Verification items for the finished model (mm, model axes). A direction names the side the tool comes from. Coordinates: 2 decimals unless noted, no trailing zeros. Order: outer loops, then holes, each group sorted by start corner. A loop starts at its lowest first (then second) coordinate and runs counter-clockwise, first axis right, second up. Notation, with made-up numbers: M 48,83 L 105,83 A11 ccw 105,90 Z; hole C 88,70 d4. An arc over 180 degrees is marked long. Return JSON: item names as keys, results as strings.
```python
from build123d import *

# Parameters (mm, degrees)
F1_DEPTH = 30
F2_R     = 2.25
F3_DEPTH = 25
F5_DEPTH = 4
F6_SIZE  = 5


with BuildPart() as f1:
    # F0 (on Top) → F1 (new body)
    with BuildSketch(Plane.XY):
        with BuildLine():
            ThreePointArc((6.4, 16.018817), (0, -17.25), (-6.4, 16.018817))
            Line((-6.4, 16.018817), (-6.4, 22.25))
            Line((-6.4, 22.25), (-44.75, 22.25))
            Line((-44.75, 22.25), (-44.75, 14.25))
            Line((-44.75, 14.25), (-22.25, 14.25))
            Line((-22.25, 14.25), (-22.25, 0))
            ThreePointArc((-22.25, 0), (0, -22.25), (22.25, 0))
            Line((22.25, 0), (22.25, 14.25))
            Line((22.25, 14.25), (44.75, 14.25))
            Line((44.75, 14.25), (44.75, 22.25))
            Line((44.75, 22.25), (6.4, 22.25))
            Line((6.4, 22.25), (6.4, 16.018817))
        make_face()
    extrude(amount=F1_DEPTH)

    # F2 (on face) → F3 (cut)
    with BuildSketch(Plane.XZ.offset(-14.25)):
        with Locations((-34.75, 22.5)):
            Circle(F2_R)
        with Locations((-34.75, 7.5)):
            Circle(F2_R)
        with Locations((34.75, 22.5)):
            Circle(F2_R)
        with Locations((34.75, 7.5)):
            Circle(F2_R)
    extrude(amount=-F3_DEPTH, mode=Mode.SUBTRACT)

    # F4 (on face) → F5 (cut)
    with BuildSketch(Plane.XZ.offset(-14.25)):
        Polygon((-30.525, 20.060695), (-30.525, 24.939305), (-34.75, 27.37861), (-38.975, 24.939305), (-38.975, 20.060695), (-34.75, 17.62139), align=None)
        Polygon((-30.525, 5.060695), (-30.525, 9.939305), (-34.75, 12.37861), (-38.975, 9.939305), (-38.975, 5.060695), (-34.75, 2.62139), align=None)
        Polygon((38.975, 5.060695), (38.975, 9.939305), (34.75, 12.37861), (30.525, 9.939305), (30.525, 5.060695), (34.75, 2.62139), align=None)
        Polygon((34.75, 27.37861), (30.525, 24.939305), (30.525, 20.060695), (34.75, 17.62139), (38.975, 20.060695), (38.975, 24.939305), align=None)
    extrude(amount=-F5_DEPTH, mode=Mode.SUBTRACT)

    # F6
    f6_edges = [f1.edges().sort_by_distance(p)[0] for p in [
        (-22.25, 14.25, 15),
        (22.25, 14.25, 15),
    ]]
    chamfer(f6_edges, length=F6_SIZE)


solid = f1.part
```
Q1. Go/stop test with flat-tipped pins: pin 1 (1.5 mm diameter, centred on y = 13, z = 16.5, fed in from -X); pin 2 (5 mm diameter, centred on y = 8.5, z = 10, fed in from +X); pin 3 (1 mm diameter, centred on x = -26.5, z = 11, fed in from -Y). Record where each tip stops, or that it passes through.
Values:
{"pin 1": "x = -26.75", "pin 2": "x = 24", "pin 3": "y = 13"}
Q2. Cross-section at D-D, the plane z = 14.75. Record the boundary of the cut face in (x, y), and give its area (3 significant figures).
Values:
{"outline": "M -44.75,14.25 L -27.25,14.25 L -22.25,9.25 L -22.25,0 A22.25 ccw 22.25,0 L 22.25,9.25 L 27.25,14.25 L 44.75,14.25 L 44.75,22.25 L 6.4,22.25 L 6.4,16.02 A17.25 cw long -6.4,16.02 L -6.4,22.25 L -44.75,22.25 Z", "area": "1,150 mm^2"}
Q3. Draft check along X on faces 1 (the face through (-33.712, 20.222, 20.504)), 2 (the face through (44.75, 18, 15)), 3 (the face through (9, 15, 0)). Enter one of: pulls with the +X half, pulls with the -X half, needs draft (parallel to the pull), parting line crosses it, or undercut.
Values:
{"face 1": "undercut", "face 2": "pulls with the +X half", "face 3": "needs draft"}
Q4. Cross-section at A-A, the plane z = 7.5. State how many separate pieces and enclosed holes the cut face has, and give its area (3 significant figures).
Values:
{"separate pieces": "3", "enclosed holes": "0", "area": "1,050 mm^2"}
Q5. Cross-section at C-C, the plane y = -15.5. Record the boundary of the cut face in (x, z), and give its area (3 significant figures).
Values:
{"outline": "M -15.96,0 L -7.57,0 L -7.57,30 L -15.96,30 Z; M 7.57,0 L 15.96,0 L 15.96,30 L 7.57,30 Z", "area": "504 mm^2"}
Q6. Cross-section at B-B, the plane x = -7.5. Record the boundary of the cut face in (y, z), and give its area (3 significant figures).
Values:
{"outline": "M -20.95,0 L -15.53,0 L -15.53,30 L -20.95,30 Z; M 15.53,0 L 22.25,0 L 22.25,30 L 15.53,30 Z", "area": "364 mm^2"}
Q7. Tool access check on faces 4 (the face through (9, 15, 30)), 5 (the face through (32.608, 16.222, 18.858)), 6 (the face through (6.4, 19, 15)). Record the directions out of +Z, -Z, +X, -X, +Y, -Y that give a thin tool (end or side, any length) a straight path to the whole face; none if there is none.
Values:
{"face 4": "+Z, +X, -X, +Y, -Y", "face 5": "-Y", "face 6": "+Z, -Z, +Y"}
Q8. Material ranges on line 1 along Z through (x, y) = (-34.75, 21.1); line 2 along X through (y, z) = (16.5, 24.5) (3 decimals); line 3 along X through (y, z) = (19, 11.75), recorded low to high.
Values:
{"line 1": "0 to 5.25, 9.75 to 20.25, 24.75 to 30", "line 2": "-44.75 to -38.975, -30.525 to -6.4, 6.4 to 30.525, 38.975 to 44.75", "line 3": "-44.75 to -6.4, 6.4 to 44.75"}
